The model under review builds one solid part; all positions refer to its coordinate system, in mm. A direction names the side the tool comes from. Round coordinates to 2 decimals unless told otherwise and drop trailing zeros. Loops run counter-clockwise (first coordinate to the right, second up) from the corner with the lowest first, then second, coordinate; pieces in that order, holes last. Notation, with made-up numbers: M 19,83.5 L 55,83.5 A9 cw 55,92.5 Z; hole C -13.75,85.5 d11. An arc over 180 degrees is marked long. Return JSON: item names as keys, results as strings. Group by question number.
Q1. Consider section A-A (z = 2.2). Count the separate pieces of the cut face and the enclosed holes in it, and give its area (3 significant figures).
Q2. Clearance check with flat-ended pins moving along their axes: pin 1 Ø5.5 at (x, y) = (0, 0) entering from +Z; pin 2 Ø1 at (x, z) = (10, 1.5) entering from -Y; pin 3 Ø1.5 at (x, z) = (-13, 1) entering from -Y; pin 4 Ø1.2 at (y, z) = (-142.5, 2) entering from +X. State where each tip first meets the part, or that it passes through.
Q3. Consider section B-B (y = -151). State the section outline as (x, z) points.
Q4. Consider section C-C (x = 26). State the section outline as (y, z) points.
Q5. To check wall thickness, follow line 1 along Y through (x, z) = (30, 1.2); line 2 along Y through (x, z) = (-2.5, 0.95); line 3 along Y through (x, z) = (18, 2.2). State the ranges of each line that lie inside material, in increasing order.
Q6. For faces 1 (the face through (-0.2, -113.1, 2)), 2 (the face through (-1, -97, 0)), list the 3-axis set-ups (+Z, -Z, +X, -X, +Y, -Y) from which the entire face can be reached by the end or side of a thin tool; tool diameter is ignored.
Q7. Draft analysis for pull direction Y (two halves, no side actions). For faces 3 (the face through (0.76, -234.99, 1.97)), 4 (the face through (17.92, -202.48, 1.97)), 5 (the face through (-1, -97, 4)), state which applies: pulls with the +Y half, pulls with the -Y half, needs draft (parallel to the pull), parting line crosses it, or undercut.
Autodesk Inventor part; units mm, degrees
ref_plane "YZ Plane" through (0, 0, 0) normal (1, 0, 0) x (0, 1, 0)
ref_plane "XZ Plane" through (0, 0, 0) normal (0, 1, 0) x (-1, 0, 0)
ref_plane "XY Plane" through (0, 0, 0) normal (0, 0, 1) x (1, 0, 0)
sketch "Sketch1" plane through (0, 0, 0) normal (0, 0, 1) x (1, 0, 0)
  arc A0 (37.4971, -0.4687) -> (-37.4971, -0.4688) centre (0, 0) ccw
  line L0 (0, 0) -> (0, -200) construction
  arc A1 (-35, -200) -> (35, -200) centre (0, -200) ccw
  circle A2 centre (0, -200) radius 4.75
  circle A3 centre (0, 0) radius 4.75
  line L1 (0, -200) -> (18.25, -200) construction
  circle A4 centre (18.25, -200) radius 2.5
  circle A5 centre (0, -200) radius 21 construction
  line L2 (0, -235) -> (0, -230) construction
  circle A6 centre (0, -230) radius 1.5
  line L3 (37.4971, -0.4687) -> (34.9973, -200.4375)
  line L4 (-37.4971, -0.4688) -> (-34.9973, -200.4375)
  line L5 (36.2472, -100.4531) -> (31.2476, -100.3906) construction
  line L6 (30.4976, -160.3859) -> (31.9976, -40.3953) construction
  circle A7 centre (31.9976, -40.3953) radius 1.5
  circle A8 centre (31.2476, -100.3906) radius 1.5
  circle A9 centre (30.4976, -160.3859) radius 1.5
  line L7 (37.5, 0) -> (32.5, 0) construction
  line L8 (0, 37.5) -> (0, 32.5) construction
  circle A10 centre (0, 32.5) radius 1.5
  circle A11 centre (32.5, 0) radius 1.5
  line L9 (35, -200) -> (30, -200) construction
  circle A12 centre (30, -200) radius 1.5
  circle A13 centre (-31.9976, -40.3953) radius 1.5
  circle A14 centre (-31.2476, -100.3906) radius 1.5
  circle A15 centre (-30.4976, -160.3859) radius 1.5
  circle A16 centre (-32.5, 0) radius 1.5
  line L10 (-35, -200) -> (-30, -200) construction
  circle A17 centre (-30, -200) radius 1.5
  line L11 (0, 0) -> (16, 0) construction
  circle A18 centre (16, 0) radius 2.5
  line L12 (0, -200) -> (-18.25, -200) construction
  circle A19 centre (-18.25, -200) radius 2.5
  line L13 (0, 0) -> (-16, 0) construction
  circle A20 centre (-16, 0) radius 2.5
  line L14 (0, -200) -> (0, -126.1) construction
  circle A21 centre (0, -126.1) radius 11 construction
  line L15 (-21, -147.1) -> (21, -147.1) construction
  line L16 (21, -147.1) -> (21, -105.1) construction
  line L17 (21, -105.1) -> (-21, -105.1) construction
  line L18 (-21, -105.1) -> (-21, -147.1) construction
  line L19 (-21, -147.1) -> (21, -105.1) construction
  line L20 (21, -147.1) -> (-8.7136, -117.3864) construction
  line L21 (0, -124.1) -> (0, -128.1) construction
  arc A22 (-11, -128.1) -> (11, -128.1) centre (0, -128.1) ccw
  line L22 (-11, -124.1) -> (-11, -128.1)
  line L23 (11, -124.1) -> (11, -128.1)
  arc A23 (11, -124.1) -> (-11, -124.1) centre (0, -124.1) ccw
  line L24 (15.5, -126.1) -> (-15.5, -126.1) construction
  line L25 (0, -141.6) -> (0, -110.6) construction
  circle A24 centre (-15.5, -110.6) radius 1.5 construction
  line L26 (-15.5, -108.6) -> (-15.5, -112.6) construction
  arc A25 (-14, -108.6) -> (-17, -108.6) centre (-15.5, -108.6) ccw
  arc A26 (-17, -112.6) -> (-14, -112.6) centre (-15.5, -112.6) ccw
  line L27 (-17, -112.6) -> (-17, -108.6)
  line L28 (-14, -112.6) -> (-14, -108.6)
  circle A27 centre (15.5, -110.6) radius 1.5 construction
  line L29 (15.5, -108.6) -> (15.5, -112.6) construction
  arc A28 (17, -108.6) -> (14, -108.6) centre (15.5, -108.6) ccw
  arc A29 (14, -112.6) -> (17, -112.6) centre (15.5, -112.6) ccw
  line L30 (17, -112.6) -> (17, -108.6)
  line L31 (14, -112.6) -> (14, -108.6)
  circle A30 centre (-15.5, -141.6) radius 1.5 construction
  line L32 (-15.5, -143.6) -> (-15.5, -139.6) construction
  arc A31 (-17, -143.6) -> (-14, -143.6) centre (-15.5, -143.6) ccw
  arc A32 (-14, -139.6) -> (-17, -139.6) centre (-15.5, -139.6) ccw
  line L33 (-17, -139.6) -> (-17, -143.6)
  line L34 (-14, -139.6) -> (-14, -143.6)
  arc A33 (14, -143.6) -> (17, -143.6) centre (15.5, -143.6) ccw
  circle A34 centre (15.5, -141.6) radius 1.5 construction
  line L35 (17, -139.6) -> (17, -143.6)
  line L36 (15.5, -143.6) -> (15.5, -139.6) construction
  arc A35 (17, -139.6) -> (14, -139.6) centre (15.5, -139.6) ccw
  line L37 (14, -139.6) -> (14, -143.6)
  dimension "D_Junta2" = 75
  dimension "L_Elo" = 200
  dimension "D_Junta3" = 70
  dimension "Veio" = 9.5
  dimension "d4" = 9.5
  dimension "d5" = 18.25
  dimension "d6" = 5
  dimension "D_P" = 42
  dimension "LF" = 5
  dimension "D_Sup" = 3
  dimension "d10" = 5
  dimension "d12" = 120
  dimension "d13" = 3
  dimension "d14" = 3
  dimension "d15" = 3
  dimension "d16" = 5
  dimension "d17" = 5
  dimension "d18" = 3
  dimension "d19" = 3
  dimension "d20" = 5
  dimension "d21" = 3
  dimension "d22" = 16
  dimension "d23" = 5
  dimension "CA" = 73.9
  dimension "DN" = 22
  dimension "d29" = 42
  dimension "d30" = 42
  dimension "NN" = 4
  dimension "d45" = 22
  dimension "d46" = 11
  dimension "d47" = 31
  dimension "d48" = 31
  dimension "FN" = 3
  dimension "d50" = 15.5
  dimension "d51" = 15.5
  dimension "d52" = 4
  dimension "d53" = 3
  dimension "d54" = 3
extrude "Extrusion1" add sketch "Sketch1" along normal blind 4
equation "\"d4\" = Veio"
equation "\"d10\" = LF"
equation "\"d13\" = D_Sup"
equation "\"d14\" = D_Sup"
equation "\"d15\" = D_Sup"
equation "\"d16\" = LF"
equation "\"d17\" = LF"
equation "\"d18\" = D_Sup"
equation "\"d19\" = D_Sup"
equation "\"d20\" = LF"
equation "\"d21\" = D_Sup"
equation "\"d45\" = DN"
equation "\"d46\" = 0.5 * DN"
equation "\"d52\" = NN"
equation "\"d53\" = FN"
equation "\"d54\" = FN"
equation "\"d44\" = DN"
properties part number "3ELO"
Values:
{
 "1": {"separate pieces": "1", "enclosed holes": "23", "area": "17,800 mm2"},
 "2": {"pin 1": "passes through", "pin 2": "stops at y = -233.69", "pin 3": "stops at y = -232.79", "pin 4": "stops at x = 35.73"},
 "3": {"outline": "M -35.62,0 L 35.62,0 L 35.62,4 L -35.62,4 Z"},
 "4": {"outline": "M -223.43,0 L 27.02,0 L 27.02,4 L -223.43,4 Z"},
 "5": {"line 1": "y = -218.03 to -201.5, -198.5 to -161.8, -158.97 to -101.22, -99.56 to 22.5", "line 2": "y = -234.91 to -204.04, -195.96 to -138.81, -113.39 to -4.04, 4.04 to 37.42", "line 3": "y = -230.02 to -202.49, -197.51 to -1.5, 1.5 to 32.9"},
 "6": {"face 1": "+Z, -Z", "face 2": "-Z, +X, -X, +Y, -Y"},
 "7": {"face 3": "pulls with the -Y half", "face 4": "undercut", "face 5": "needs draft"}
}
